Could you check a few things on this model? Use its own coordinates, in mm. Face numbers are marked on the shaded views. A direction names the side the tool comes from. Coordinates: 2 decimals unless noted, no trailing zeros. Write each loop counter-clockwise with the first axis right and the second up, starting at its lowest first coordinate (ties: lowest second). Pieces come first, ordered by that corner, then holes. Notation, with made-up numbers: M 62,84 L 107,84 A17 cw 107,91 Z; hole C 69,52 d4. An arc over 180 degrees is marked long. Answer as CSV lines item,"result". Start each with the question number.
Item 1: Suppose I cut it at B-B, the plane z = 1.5. Write out the boundary of the cut face in (x, y).
Item 2: If I drill on line 1 along X through (y, z) = (1.1, 1.5); line 2 along Z through (x, y) = (6.7, 1.7); line 3 along X through (y, z) = (-0.85, 1.5), over which ranges is the centre line in solid material (lowest first)? Write a range as [from, to].
Item 3: On a 3-axis mill with a long thin cutter (end or side, diameter ignored), from which of +Z, -Z, +X, -X, +Y, -Y can I reach the whole of each face in a straight line? I mean the marked faces 1 and 2. Say none if no direction works.
Item 4: Suppose I cut it at C-C, the plane y = 1.65. Write out the boundary of the cut face in (x, z).
Item 5: Suppose I cut it at D-D, the plane x = 4. Write out the boundary of the cut face in (y, z).
Item 6: I'm going to push flat-ended pins straight in: P1, Ø1.5, axis at x = 5.5, z = 1, coming from the +Y side; P2, Ø1.5, axis at x = 1, z = 2, coming from the -Y side; P3, Ø1, axis at x = 5.5, z = 0.5, coming from the +Y side. Where does each tip first touch, or does it pass through?
Item 7: Suppose I cut it at A-A, the plane x = 1. Write out the boundary of the cut face in (y, z), and give its area (3 significant figures).
```python
from build123d import *
from OCP.BRepFilletAPI import BRepFilletAPI_MakeChamfer
from build123d.topology import SkipClean

# Parameters (mm, degrees)
SKETCH1_W           = 8
SKETCH1_H           = 3
BOSS_EXTRUDE1_DEPTH = 2.2
SKETCH2_R           = 1
BOSS_EXTRUDE2_DEPTH = 0.6
SKETCH3_R           = 0.5
CUT_EXTRUDE1_DEPTH  = 2.5
SKETCH4_W           = 5.5
SKETCH4_H           = 3
BOSS_EXTRUDE3_DEPTH = 2.2
BOSS_EXTRUDE4_START = 0.6
SKETCH5_R           = 1
BOSS_EXTRUDE4_DEPTH = 0.6
CUT_EXTRUDE2_START  = -2.5
SKETCH6_R           = 0.5
CUT_EXTRUDE2_DEPTH  = 2.5
CHAMFER1_SIZE       = 0.25
CHAMFER1_SIZE2      = 0.433012702
FILLET1_R           = 0.5
CHAMFER2_SIZE       = 0.3
CHAMFER2_SIZE2      = 0.519615242


with BuildPart() as part:
    # Sketch1 → Boss-Extrude1 (new body)
    with BuildSketch(Plane(origin=(0, 0, 0), x_dir=(1, 0, 0), z_dir=(0, 1, 0))):
        with Locations((4, -1.5)):
            Rectangle(SKETCH1_W, SKETCH1_H)
    extrude(amount=BOSS_EXTRUDE1_DEPTH)

    # Sketch2 → Boss-Extrude2 (add)
    with BuildSketch(Plane(origin=(0, 2.2, 0), x_dir=(1, 0, 0), z_dir=(0, 1, 0))):
        with Locations(Location((4, -1.5, 0), (0, 0, 270))):
            Circle(SKETCH2_R)
    extrude(amount=BOSS_EXTRUDE2_DEPTH)

    # Sketch3 → Cut-Extrude1 (cut)
    with BuildSketch(Plane(origin=(0, 2.2, 0), x_dir=(1, 0, 0), z_dir=(0, 1, 0))):
        with Locations(Location((1.3, -1.5, 0), (0, 0, 270))):
            Circle(SKETCH3_R)
        with Locations(Location((6.7, -1.5, 0), (0, 0, 270))):
            Circle(SKETCH3_R)
    extrude(amount=-CUT_EXTRUDE1_DEPTH, mode=Mode.SUBTRACT)

    # Sketch4 → Boss-Extrude3 (add)
    with BuildSketch(Plane.XZ):
        with Locations((5.25, 1.5)):
            Rectangle(SKETCH4_W, SKETCH4_H)
    extrude(amount=BOSS_EXTRUDE3_DEPTH)

    # Sketch5 → Boss-Extrude4 (add)
    with BuildSketch(Plane.XZ.offset(2.2).offset(BOSS_EXTRUDE4_START)):
        with Locations(Location((4, 1.5, 0), (0, 0, 90))):
            Circle(SKETCH5_R)
    extrude(amount=-BOSS_EXTRUDE4_DEPTH)

    # Sketch6 → Cut-Extrude2 (cut)
    with SkipClean():  # the faces are left unmerged after this step: merging them gives an invalid solid
        with BuildSketch(Plane.XZ.offset(2.2).offset(CUT_EXTRUDE2_START)):
            with Locations(Location((6.7, 1.5, 0), (0, 0, 270))):
                Circle(SKETCH6_R)
        extrude(amount=CUT_EXTRUDE2_DEPTH, mode=Mode.SUBTRACT)

    # Chamfer1: one chamfer whose edges measure the first distance from different faces: ONE call of the kernel's chamfer builder (chamfer() names one face for all edges)
    chamfer1_edges_1 = [part.edges().sort_by_distance(p)[0] for p in [
        (1.25, 0, 0),
        (2.5, -1.1, 0),
        (0, 1.1, 0),
        (8, 0, 0),
    ]]
    chamfer1_side_1 = [part.faces().sort_by_distance(p)[0] for p in [
        (4.509259259, 0.203703704, 0),
    ]]
    chamfer1_edges_2 = [part.edges().sort_by_distance(p)[0] for p in [
        (2.5, -1.1, 3),
        (1.25, 0, 3),
        (8, 0, 3),
        (0, 1.1, 3),
    ]]
    chamfer1_side_2 = [part.faces().sort_by_distance(p)[0] for p in [
        (4.509259259, 0.203703704, 3),
    ]]
    chamfer1 = BRepFilletAPI_MakeChamfer(part.part.solid().wrapped)
    for e in chamfer1_edges_1:
        chamfer1.Add(CHAMFER1_SIZE, CHAMFER1_SIZE2, e.wrapped, chamfer1_side_1[0].wrapped)  # the first distance lies on this face
    for e in chamfer1_edges_2:
        chamfer1.Add(CHAMFER1_SIZE, CHAMFER1_SIZE2, e.wrapped, chamfer1_side_2[0].wrapped)  # the first distance lies on this face
    add(Compound.cast(chamfer1.Shape()), mode=Mode.REPLACE)

    # Fillet1
    fillet1_edges = [part.edges().sort_by_distance(p)[0] for p in [
        (8, 0, 2.566987298),
        (8, 0, 0.433012702),
        (2.5, -1.1, 2.566987298),
        (2.5, -1.1, 0.433012702),
        (1.25, 0, 2.566987298),
        (1.25, 0, 0.433012702),
        (0, 1.1, 2.566987298),
        (0, 1.1, 0.433012702),
    ]]
    fillet(fillet1_edges, radius=FILLET1_R)

    # Chamfer2: one chamfer whose edges measure the first distance from different faces: ONE call of the kernel's chamfer builder (chamfer() names one face for all edges)
    chamfer2_edges_1 = [part.edges().sort_by_distance(p)[0] for p in [
        (4, 2.8, 0.5),
    ]]
    chamfer2_side_1 = [part.faces().sort_by_distance(p)[0] for p in [
        (4, 2.5, 0.5),
    ]]
    chamfer2_edges_2 = [part.edges().sort_by_distance(p)[0] for p in [
        (4, -2.8, 0.5),
    ]]
    chamfer2_side_2 = [part.faces().sort_by_distance(p)[0] for p in [
        (4, -2.5, 0.5),
    ]]
    chamfer2 = BRepFilletAPI_MakeChamfer(part.part.solid().wrapped)
    for e in chamfer2_edges_1:
        chamfer2.Add(CHAMFER2_SIZE, CHAMFER2_SIZE2, e.wrapped, chamfer2_side_1[0].wrapped)  # the first distance lies on this face
    for e in chamfer2_edges_2:
        chamfer2.Add(CHAMFER2_SIZE, CHAMFER2_SIZE2, e.wrapped, chamfer2_side_2[0].wrapped)  # the first distance lies on this face
    add(Compound.cast(chamfer2.Shape()), mode=Mode.REPLACE)


solid = part.part
```
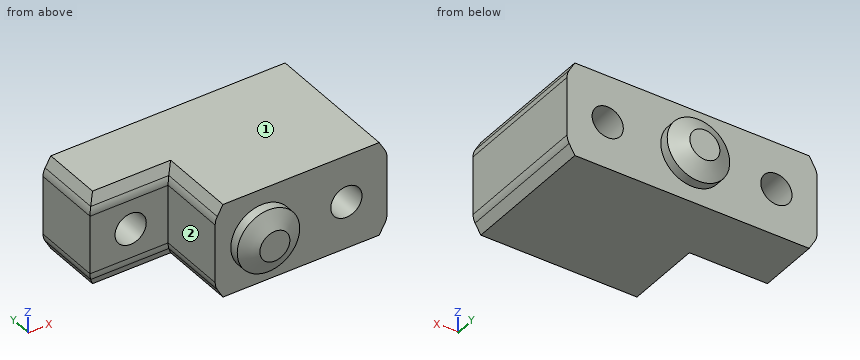
Ans:
1,outline,"M 0,0 L 0.8,0 L 0.8,2.2 L 0,2.2 Z; M 1.8,0 L 2.5,0 L 2.5,-2.2 L 3,-2.2 L 3,-2.5 L 3.52,-2.8 L 4.48,-2.8 L 5,-2.5 L 5,-2.2 L 6.2,-2.2 L 6.2,2.2 L 5,2.2 L 5,2.5 L 4.48,2.8 L 3.52,2.8 L 3,2.5 L 3,2.2 L 1.8,2.2 Z; M 7.2,-2.2 L 8,-2.2 L 8,2.2 L 7.2,2.2 Z"
2,line 1,"x = [0, 0.8], [1.8, 6.2], [7.2, 8]"
2,line 2,"z = [0, 1], [2, 3]"
2,line 3,"x = [2.5, 6.2], [7.2, 8]"
3,face 1,"+Z, +X, -X, +Y, -Y"
3,face 2,"+Z, -Z, -X, -Y"
4,outline,"M 0,0.57 A0.5 ccw 0.07,0.32 L 0.25,0 L 7.75,0 L 7.93,0.32 A0.5 ccw 8,0.57 L 8,2.43 A0.5 ccw 7.93,2.68 L 7.75,3 L 0.25,3 L 0.07,2.68 A0.5 ccw 0,2.43 Z; hole C 1.3,1.5 d1; hole C 6.7,1.5 d1"
5,outline,"M -2.8,1.02 L -2.5,0.5 L -2.2,0.5 L -2.2,0 L 2.2,0 L 2.2,0.5 L 2.5,0.5 L 2.8,1.02 L 2.8,1.98 L 2.5,2.5 L 2.2,2.5 L 2.2,3 L -2.2,3 L -2.2,2.5 L -2.5,2.5 L -2.8,1.98 Z"
6,P1,"stops at y = 2.6"
6,P2,"stops at y = 0"
6,P3,"stops at y = 2.2"
7,outline,"M 0,0.57 A0.5 ccw 0.07,0.32 L 0.25,0 L 2.2,0 L 2.2,1.1 L 0,1.1 Z; M 0,1.9 L 2.2,1.9 L 2.2,3 L 0.25,3 L 0.07,2.68 A0.5 ccw 0,2.43 Z"
7,area,"4.73 mm^2"
